For this review, take the finished solid that the model builds, in its own axes (mm). A direction names the side the tool comes from. Round coordinates to 2 decimals unless told otherwise and drop trailing zeros. Order: outer loops, then holes, each group sorted by start corner. A loop starts at its lowest first (then second) coordinate and runs counter-clockwise, first axis right, second up.
from build123d import *

# Parameters (mm, degrees)
SKETCH1_R           = 75
BOSS_EXTRUDE1_DEPTH = 105
SKETCH3_R           = 51
BOSS_EXTRUDE3_DEPTH = 102
BOSS_EXTRUDE4_START = -105
SKETCH7_R           = 75
BOSS_EXTRUDE4_DEPTH = 105
BOSS_EXTRUDE5_START = -180
SKETCH8_R           = 38
BOSS_EXTRUDE5_DEPTH = 75


with BuildPart() as part:
    # Sketch1 → Boss-Extrude1 (new body)
    with BuildSketch(Plane.XY):
        with BuildLine():
            Line((495, -355), (495, 355))
            Line((495, 355), (220, 355))
            Line((220, 355), (-98.810385884, 179.614887026))
            ThreePointArc((-98.810385884, 179.614887026), (-205, 0), (-98.810385884, -179.614887026))
            Line((-98.810385884, -179.614887026), (220, -355))
            Line((220, -355), (495, -355))
        make_face()
        Circle(SKETCH1_R, mode=Mode.SUBTRACT)
    extrude(amount=-BOSS_EXTRUDE1_DEPTH)

    # Sketch3 → Boss-Extrude3 (add)
    with BuildSketch(Plane(origin=(0, 355, 0), x_dir=(1, 0, 0), z_dir=(0, 1, 0))):
        with BuildLine():
            ThreePointArc((900.990279967, 165.185790909), (908.113739275, 56.502804044), (815, 0))
            Line((815, 0), (495, 0))
            Line((495, 0), (495, 105))
            Line((495, 105), (220, 105))
            Line((220, 105), (220, 745))
            Line((220, 745), (495, 745))
            Line((495, 745), (900.990279967, 165.185790909))
        make_face()
        with Locations(Location((815, 104.974748664, 0), (0, 0, 180))):
            Circle(SKETCH3_R, mode=Mode.SUBTRACT)
    boss_extrude3 = extrude(amount=-BOSS_EXTRUDE3_DEPTH)

    # Mirror1: Boss-Extrude3 across plane
    add(boss_extrude3.mirror(Plane.ZX))

    # Sketch7 → Boss-Extrude4 (add)
    with BuildSketch(Plane(origin=(0, 0, -745), x_dir=(-1, 0, 0), z_dir=(0, 0, -1)).offset(BOSS_EXTRUDE4_START)):
        with BuildLine():
            Line((-220, -253), (-220, -355))
            Line((-220, -355), (98.810385884, -179.614887026))
            ThreePointArc((98.810385884, -179.614887026), (205, 0), (98.810385884, 179.614887026))
            Line((98.810385884, 179.614887026), (-220, 355))
            Line((-220, 355), (-495, 355))
            Line((-495, 355), (-495, -253))
            Line((-495, -253), (-220, -253))
        make_face()
        with Locations(Location((0, 0, 0), (0, 0, 180))):
            Circle(SKETCH7_R, mode=Mode.SUBTRACT)
    extrude(amount=BOSS_EXTRUDE4_DEPTH)

    # Sketch8 → Boss-Extrude5 (add)
    with BuildSketch(Plane(origin=(0, 355, 0), x_dir=(1, 0, 0), z_dir=(0, 1, 0)).offset(BOSS_EXTRUDE5_START)):
        with BuildLine():
            Line((440.558080551, 1007.850884872), (220, 745))
            Line((220, 745), (454.97331208, 745))
            Line((454.97331208, 745), (578.446080312, 892.149115128))
            ThreePointArc((578.446080312, 892.149115128), (567.352965303, 1018.943999881), (440.558080551, 1007.850884872))
        make_face()
        with Locations(Location((509.502080431, 950, 0), (0, 0, 180))):
            Circle(SKETCH8_R, mode=Mode.SUBTRACT)
    boss_extrude5 = extrude(amount=-BOSS_EXTRUDE5_DEPTH)

    # Mirror2: Boss-Extrude5 across plane
    add(boss_extrude5.mirror(Plane.ZX))


solid = part.part
(1) Add section D-D on x = 353. Give the boundary of the cut face in (y, z).
(2) Add section C-C on x = 691.5. Give the boundary of the cut face in (y, z).
(3) Add section B-B on z = -420. Give the boundary of the cut face in (x, y).
(4) Wall thickness on L1, parallel to Y at x = 386, z = -792.5; L2, parallel to Z at x = 75, y = 162.5; L3, parallel to Z at x = 815, y = -280: over which ranges is each line inside the solid? List them lowest first.
(5) Draft analysis for pull direction X (two halves, no side actions). For faces 6 (the face through (449, 100, -862)), 7 (the face through (491.967, -138.025, -983.713)), 8 (the face through (58.4, 266.1, -691.8)), state which applies: pulls with the +X half, pulls with the -X half, needs draft (parallel to the pull), parting line crosses it, or undercut.
(6) Clearance check with flat-ended pins moving along their axes: P1, Ø1.5, axis at x = -8.5, z = -740, coming from the -Y side; P2, Ø4, axis at x = 149.5, y = 67, coming from the -Z side; P3, Ø5, axis at x = 196.5, z = -702.5, coming from the +Y side. State where each tip first meets the part, or that it passes through.
(7) Add section A-A on y = 0. Give the boundary of the cut face in (x, z).
(8) Tool access review of faces 1 (the face through (695.153, -304.714, -459.152)), 2 (the face through (515.845, 138.025, -817.545)), 3 (the face through (58.4, -266.1, -51.8)), 4 (the face through (497, 253, -295)), 5 (the face through (449, 175, -862)): name each direction out of +Z, -Z, +X, -X, +Y, -Y from which nothing blocks a thin tool from reaching the whole face with its end or side.
Here are the results:
1. outline: (-355, -745) - (-175, -745) - (-175, -903.5) - (-100, -903.5) - (-100, -745) - (100, -745) - (100, -903.5) - (175, -903.5) - (175, -745) - (355, -745) - (355, 0) - (-355, 0) - close; hole (-253, -640) - (253, -640) - (253, -105) - (-253, -105) - close
2. outline: (-355, -464.37) - (-253, -464.37) - (-253, 0) - (-355, 0) - close; (253, -464.37) - (355, -464.37) - (355, 0) - (253, 0) - close
3. outline: (220, -355) - (722.57, -355) - (722.57, -253) - (220, -253) - close; (220, 253) - (722.57, 253) - (722.57, 355) - (220, 355) - close
4. L1: y = -175 to -100, 100 to 175
4. L2: z = -745 to -640, -105 to 0
4. L3: z = -287.99 to -155.97, -53.97 to 0
5. face 6: needs draft
5. face 7: undercut
5. face 8: pulls with the -X half
6. P1: stops at y = -229.71
6. P2: stops at z = -745
6. P3: stops at y = 343.45
7. outline: (-205, -745) - (-75, -745) - (-75, -640) - (-205, -640) - close; (-205, -105) - (-75, -105) - (-75, 0) - (-205, 0) - close; (75, -745) - (495, -745) - (495, -640) - (75, -640) - close; (75, -105) - (495, -105) - (495, 0) - (75, 0) - close
8. face 1: -Z, +X, +Y, -Y
8. face 2: +X, +Y, -Y
8. face 3: +Z, -Z, -X, -Y
8. face 4: +X
8. face 5: -Z, +X, -X, +Y
